Input: part model. Units: mm. Frame: model coordinates. A direction names the side the tool comes from. Give positions to 0.01 mm unless a question says otherwise; leave off trailing zeros. Loops run counter-clockwise (first coordinate to the right, second up) from the corner with the lowest first, then second, coordinate; pieces in that order, holes last. Notation, with made-up numbers: (29, -6.75) -> (82, -6.75) arc R30 cw to (82, 19.25) -> close; hole circle Ø6 at (88.5, 23.25). An arc over 180 degrees is marked (long way). Answer in a Markdown table with one row per item. Add a question column.
```python
from build123d import *

# Parameters (mm, degrees)
F1_DEPTH = 1371.6
F2_R     = 25.4
F3_DEPTH = 6.35
F4_R     = 25.4
F5_DEPTH = 6.35


with BuildPart() as f1:
    # F0 (on Top) → F1 (new body)
    with BuildSketch(Plane.XY):
        with BuildLine():
            Line((44.45, 50.8), (-44.45, 50.8))
            ThreePointArc((-44.45, 50.8), (-48.940128, 48.940128), (-50.8, 44.45))
            Line((-50.8, 44.45), (-50.8, -44.45))
            ThreePointArc((-50.8, -44.45), (-48.940128, -48.940128), (-44.45, -50.8))
            Line((-44.45, -50.8), (44.45, -50.8))
            ThreePointArc((44.45, -50.8), (48.940128, -48.940128), (50.8, -44.45))
            Line((50.8, -44.45), (50.8, 44.45))
            ThreePointArc((50.8, 44.45), (48.940128, 48.940128), (44.45, 50.8))
        make_face()
        with BuildLine():
            ThreePointArc((-44.45, 41.275), (-43.520064, 43.520064), (-41.275, 44.45))
            Line((-41.275, 44.45), (41.275, 44.45))
            ThreePointArc((41.275, 44.45), (43.520064, 43.520064), (44.45, 41.275))
            Line((44.45, 41.275), (44.45, -41.275))
            ThreePointArc((44.45, -41.275), (43.520064, -43.520064), (41.275, -44.45))
            Line((41.275, -44.45), (-41.275, -44.45))
            ThreePointArc((-41.275, -44.45), (-43.520064, -43.520064), (-44.45, -41.275))
            Line((-44.45, -41.275), (-44.45, 41.275))
        make_face(mode=Mode.SUBTRACT)
    extrude(amount=F1_DEPTH)

    # F2 (on face) → F3 (cut, through all)
    with BuildSketch(Plane(origin=(0, 50.8, 0), x_dir=(-1, 0, 0), z_dir=(0, 1, 0))):
        with Locations((0, 644.525)):
            Circle(F2_R)
        with Locations((0, 44.45)):
            Circle(F2_R)
    extrude(amount=-F3_DEPTH, mode=Mode.SUBTRACT)

    # F4 (on face) → F5 (cut, through all)
    with BuildSketch(Plane.XZ.offset(50.8)):
        with Locations((0, 1101.725)):
            Circle(F4_R)
    extrude(amount=-F5_DEPTH, mode=Mode.SUBTRACT)


solid = f1.part
```
1) Section C-C on y = -11. Output: boundary loops of the cut face in (x, z).
2) Material intervals for line 1 along Z through (x, y) = (0, 46) (3 decimals); line 2 along Y through (x, z) = (35.5, 385.5), sorted ascending.
3) Pull-direction query (X, two-part tool) for faces 1 (the face through (50.8, -1, 676)), 2 (the face through (5.51, 47.67, 619.73)), 3 (the face through (-1, -50.8, 676)); classes: +X half, -X half, draft (parallel to the pull), parting line (faces both ways), or undercut.
4) Section B-B on z = 86. Output: boundary loops of the cut face in (x, y) (3 decimals), and give its area (3 significant figures).
5) Section A-A on x = 0. Output: boundary loops of the cut face in (y, z) (3 decimals).
6) Reachability of faces 4 (the face through (4, -45, 0)), 5 (the face through (-3.31, -47.67, 1126.91)), 6 (the face through (5.506, 47.669, 19.654)), 7 (the face through (-44.45, -1, 676)), 8 (the face through (1, 50.8, 676)) from +Z, -Z, +X, -X, +Y, -Y: full face, straight path, thin tool, end or side. Return the list, or none.
Working result:
| question | item | result |
|---|---|---|
| 1 | outline | (-50.8, 0) -> (-44.45, 0) -> (-44.45, 1371.6) -> (-50.8, 1371.6) -> close; (44.45, 0) -> (50.8, 0) -> (50.8, 1371.6) -> (44.45, 1371.6) -> close |
| 2 | line 1 | z = 0 to 19.05, 69.85 to 619.125, 669.925 to 1371.6 |
| 2 | line 2 | y = -50.8 to -44.45, 44.45 to 50.8 |
| 3 | face 1 | +X half |
| 3 | face 2 | undercut |
| 3 | face 3 | draft |
| 4 | outline | (-50.8, -44.45) arc R6.35 ccw to (-44.45, -50.8) -> (44.45, -50.8) arc R6.35 ccw to (50.8, -44.45) -> (50.8, 44.45) arc R6.35 ccw to (44.45, 50.8) -> (-44.45, 50.8) arc R6.35 ccw to (-50.8, 44.45) -> close; hole (-44.45, -41.275) arc R3.175 ccw to (-41.275, -44.45) -> (41.275, -44.45) arc R3.175 ccw to (44.45, -41.275) -> (44.45, 41.275) arc R3.175 ccw to (41.275, 44.45) -> (-41.275, 44.45) arc R3.175 ccw to (-44.45, 41.275) -> close |
| 4 | area | 2,390 mm2 |
| 5 | outline | (-50.8, 0) -> (-44.45, 0) -> (-44.45, 1076.325) -> (-50.8, 1076.325) -> close; (-50.8, 1127.125) -> (-44.45, 1127.125) -> (-44.45, 1371.6) -> (-50.8, 1371.6) -> close; (44.45, 0) -> (50.8, 0) -> (50.8, 19.05) -> (44.45, 19.05) -> close; (44.45, 69.85) -> (50.8, 69.85) -> (50.8, 619.125) -> (44.45, 619.125) -> close; (44.45, 669.925) -> (50.8, 669.925) -> (50.8, 1371.6) -> (44.45, 1371.6) -> close |
| 6 | face 4 | -Z, +X, -X, +Y, -Y |
| 6 | face 5 | -Y |
| 6 | face 6 | +Y |
| 6 | face 7 | +Z, -Z |
| 6 | face 8 | +Z, -Z, +X, -X, +Y |
